from build123d import *

# Parameters (mm, degrees)
F0_R     = 50.513701
F1_DEPTH = 12.7
F2_R     = 12.303799
F3_DEPTH = 51.054
F4_R     = 29.597437
F5_DEPTH = 3.048


with BuildPart() as f1:
    # F0 (on Front) → F1 (new body)
    with BuildSketch(Plane.XZ):
        Circle(F0_R)
    extrude(amount=F1_DEPTH)

    # F2 (on Right) → F3 (join)
    with BuildSketch(Plane.YZ):
        with Locations((-5.813534, 40.69474)):
            Circle(F2_R)
    extrude(amount=F3_DEPTH)

    # F4 (on Front) → F5 (join)
    with BuildSketch(Plane.XZ):
        Circle(F4_R)
    extrude(amount=-F5_DEPTH)


solid = f1.part
Geometry: final body of the model. Coordinates: model frame, mm. A direction names the side the tool comes from. Round coordinates to 2 decimals unless told otherwise and drop trailing zeros. Loops run counter-clockwise (first coordinate to the right, second up) from the corner with the lowest first, then second, coordinate; pieces in that order, holes last.
Q1. Pull-direction query (Z, two-part tool) for faces 4 (the cylindrical face through (-6.416, 1.503, -28.894)), 5 (the flat face through (0, 3.048, 0)); classes: released by +Z, released by -Z, zero draft, split by the parting line, or undercut.
Q2. Access query for faces 1 (the flat face through (51.054, -6, 41)), 2 (the flat face through (0, 1, 43)), 3 (the flat face through (22, 0, -22)). Directions: +Z, -Z, +X, -X, +Y, -Y. A direction counts if a zero-diameter tool reaches every point of the face in a straight line with its end or side. Return the directions, or none.
Q3. Material intervals for L1, parallel to Y at x = 37.5, z = 15; L2, parallel to X at y = -15, z = 44; L3, parallel to Y at x = -15, z = 19, sorted ascending.
Q4. Section C-C on y = -1.5. Return loops of the section in (x, z).
Q5. Section D-D on x = 42. Return loops of the section in (y, z).
Q6. Section A-A on z = 0. Return loops of the section in (x, y), plus the area to 3 significant figures.
Q7. Section B-B on x = 12. Return loops of the section in (y, z), plus the area to 3 significant figures.
Q8. Pin query (flat end, axial travel): P1, Ø3, axis at y = -12.5, z = 41, coming from the -X side; P2, Ø5, axis at x = 39.5, y = -10, coming from the -Z side; P3, Ø1.5, axis at y = -1.5, z = -32, coming from the -X side. Return the tip coordinate at first contact, or that it passes through.
Evaluation:
1. face 4: undercut
1. face 5: zero draft
2. face 1: +Z, -Z, +X, +Y, -Y
2. face 2: +Z, -X
2. face 3: +Y
3. L1: y = -12.7 to 0
3. L2: x = 0 to 51.05
3. L3: y = -12.7 to 3.05
4. outline: (0, 50.51) arc R50.51 ccw (long way) to (41.24, 29.17) - (51.05, 29.17) - (51.05, 52.22) - (0, 52.22) - close
5. outline: circle Ø24.61 at (-5.81, 40.69); (-12.7, -28.06) - (0, -28.06) - (0, 28.06) - (-12.7, 28.06) - close
6. outline: (-50.51, -12.7) - (50.51, -12.7) - (50.51, 0) - (29.6, 0) - (29.6, 3.05) - (-29.6, 3.05) - (-29.6, 0) - (-50.51, 0) - close
6. area: 1,460 mm2
7. outline: (-12.7, -49.07) - (0, -49.07) - (0, -27.06) - (3.05, -27.06) - (3.05, 27.06) - (0, 27.06) - (0, 29.85) arc R12.3 ccw (long way) to (-12.7, 30.5) - close
7. area: 1,630 mm2
8. P1: stops at x = -31.49
8. P2: stops at z = -34.39
8. P3: stops at x = -39.69
